```python
from build123d import *

# Parameters (mm, degrees)
SKETCH_1_W          = 147
SKETCH_1_H          = 50
SKETCH_1_R          = 1.5
EXTRUDE_1_DEPTH     = 2
CUT_EXTRUDE_1_DEPTH = 2
FILLET_2_DEPTH      = 2
FILLET_3_R          = 4
CUT_EXTRUDE_3_DEPTH = 78.661122835
SKETCH_7_R          = 1.75
CUT_EXTRUDE_4_DEPTH = 78.661122835
FILLET_4_R          = 10


with BuildPart() as part:
    # 草图1 → 凸台-拉伸1 (new body)
    with BuildSketch(Plane(origin=(0, 0, 0), x_dir=(1, 0, 0), z_dir=(0, 1, 0))):
        Rectangle(SKETCH_1_W, SKETCH_1_H)
        with Locations(Location((18, -18, 0), (0, 0, 270))):
            Circle(SKETCH_1_R, mode=Mode.SUBTRACT)
        with Locations(Location((-18, -18, 0), (0, 0, 270))):
            Circle(SKETCH_1_R, mode=Mode.SUBTRACT)
        with Locations(Location((-18, 18, 0), (0, 0, 270))):
            Circle(SKETCH_1_R, mode=Mode.SUBTRACT)
        with Locations(Location((18, 18, 0), (0, 0, 270))):
            Circle(SKETCH_1_R, mode=Mode.SUBTRACT)
    extrude(amount=EXTRUDE_1_DEPTH)

    # 草图3 → 切除-拉伸1 (cut)
    with BuildSketch(Plane(origin=(0, 2, 0), x_dir=(1, 0, 0), z_dir=(0, 1, 0))):
        with BuildLine():
            Line((-13.345416088, 16.173843213), (0, 2.828427125))
            Line((0, 2.828427125), (13.345416088, 16.173843213))
            ThreePointArc((13.345416088, 16.173843213), (13.868972045, 20.816843629), (18, 23))
            Line((18, 23), (-18, 23))
            ThreePointArc((-18, 23), (-14.464466094, 21.535533906), (-13, 18))
            ThreePointArc((-13, 18), (-13.087112888, 17.070731352), (-13.345416088, 16.173843213))
        make_face()
        with BuildLine():
            Line((16.173843213, 13.345416088), (2.828427125, 0))
            Line((2.828427125, 0), (16.173843213, -13.345416088))
            ThreePointArc((16.173843213, -13.345416088), (20.816843629, -13.868972045), (23, -18))
            Line((23, -18), (23, 18))
            ThreePointArc((23, 18), (20.816843629, 13.868972045), (16.173843213, 13.345416088))
        make_face()
        with BuildLine():
            Line((0, -2.828427125), (-13.345416088, -16.173843213))
            ThreePointArc((-13.345416088, -16.173843213), (-13.087112888, -17.070731352), (-13, -18))
            ThreePointArc((-13, -18), (-14.464466094, -21.535533906), (-18, -23))
            Line((-18, -23), (18, -23))
            ThreePointArc((18, -23), (13.868972045, -20.816843629), (13.345416088, -16.173843213))
            Line((13.345416088, -16.173843213), (0, -2.828427125))
        make_face()
        with BuildLine():
            ThreePointArc((-23, -18), (-20.816843629, -13.868972045), (-16.173843213, -13.345416088))
            Line((-16.173843213, -13.345416088), (-2.828427125, 0))
            Line((-2.828427125, 0), (-16.173843213, 13.345416088))
            ThreePointArc((-16.173843213, 13.345416088), (-20.816843629, 13.868972045), (-23, 18))
            Line((-23, 18), (-23, -18))
        make_face()
    extrude(amount=-CUT_EXTRUDE_1_DEPTH, mode=Mode.SUBTRACT)

    # 圆角2: read off the stored shape, not the designer's step
    # 圆角2 outline → 圆角2 (add)
    with BuildSketch(Plane(origin=(0, 0, 0), x_dir=(1, 0, 0), z_dir=(0, 1, 0))):
        with BuildLine():
            Line((-23, 18), (-23, 9.05572809))
            ThreePointArc((-23, 9.05572809), (-21.666666667, 12.03715206), (-18.555555556, 13.03096005))
            ThreePointArc((-18.555555556, 13.03096005), (-21.726779962, 14.666666667), (-23, 18))
        make_face()
        with BuildLine():
            ThreePointArc((-18.555555556, -13.03096005), (-21.666666667, -12.03715206), (-23, -9.05572809))
            Line((-23, -9.05572809), (-23, -18))
            ThreePointArc((-23, -18), (-21.726779962, -14.666666667), (-18.555555556, -13.03096005))
        make_face()
        with BuildLine():
            ThreePointArc((13.03096005, -18.555555556), (12.03715206, -21.666666667), (9.05572809, -23))
            Line((9.05572809, -23), (18, -23))
            ThreePointArc((18, -23), (14.666666667, -21.726779962), (13.03096005, -18.555555556))
        make_face()
        with BuildLine():
            ThreePointArc((-9.05572809, -23), (-12.03715206, -21.666666667), (-13.03096005, -18.555555556))
            ThreePointArc((-13.03096005, -18.555555556), (-14.666666667, -21.726779962), (-18, -23))
            Line((-18, -23), (-9.05572809, -23))
        make_face()
        with BuildLine():
            ThreePointArc((18.555555556, 13.03096005), (21.666666667, 12.03715206), (23, 9.05572809))
            Line((23, 9.05572809), (23, 18))
            ThreePointArc((23, 18), (21.726779962, 14.666666667), (18.555555556, 13.03096005))
        make_face()
        with BuildLine():
            ThreePointArc((23, -9.05572809), (21.666666667, -12.03715206), (18.555555556, -13.03096005))
            ThreePointArc((18.555555556, -13.03096005), (21.726779962, -14.666666667), (23, -18))
            Line((23, -18), (23, -9.05572809))
        make_face()
        with BuildLine():
            ThreePointArc((-13.03096005, 18.555555556), (-12.03715206, 21.666666667), (-9.05572809, 23))
            Line((-9.05572809, 23), (-18, 23))
            ThreePointArc((-18, 23), (-14.666666667, 21.726779962), (-13.03096005, 18.555555556))
        make_face()
        with BuildLine():
            ThreePointArc((9.05572809, 23), (12.03715206, 21.666666667), (13.03096005, 18.555555556))
            ThreePointArc((13.03096005, 18.555555556), (14.666666667, 21.726779962), (18, 23))
            Line((18, 23), (9.05572809, 23))
        make_face()
    extrude(amount=FILLET_2_DEPTH)

    # 圆角3
    fillet_3_edges = [part.edges().sort_by_distance(p)[0] for p in [
        (13.345416088, 1, 16.173843213),
        (-13.345416088, 1, 16.173843213),
        (0, 1, 2.828427125),
        (16.173843213, 1, -13.345416088),
        (16.173843213, 1, 13.345416088),
        (2.828427125, 1, 0),
        (-16.173843213, 1, -13.345416088),
        (-2.828427125, 1, 0),
        (-16.173843213, 1, 13.345416088),
        (-13.345416088, 1, -16.173843213),
        (13.345416088, 1, -16.173843213),
        (0, 1, -2.828427125),
    ]]
    fillet(fillet_3_edges, radius=FILLET_3_R)

    # 草图6 → 切除-拉伸3 (cut, through all)
    with BuildSketch(Plane(origin=(0, 2, 0), x_dir=(1, 0, 0), z_dir=(0, 1, 0))):
        Polygon((63.5, -25), (56.57179677, -13), (36.57179677, -13), (29.643593539, -25), align=None)
    cut_extrude_3 = extrude(amount=-CUT_EXTRUDE_3_DEPTH, mode=Mode.SUBTRACT)

    # 镜向1: 切除-拉伸3 across plane
    add(cut_extrude_3.mirror(Plane(origin=(0, 0, 0), x_dir=(0, 0, 1), z_dir=(1, 0, 0))), mode=Mode.SUBTRACT)

    # 草图7 → 切除-拉伸4 (cut, through all)
    with BuildSketch(Plane.XZ):
        with Locations(Location((70.5, 20, 0), (0, 0, 270))):
            Circle(SKETCH_7_R)
        with Locations(Location((70.5, -15, 0), (0, 0, 270))):
            Circle(SKETCH_7_R)
        with Locations(Location((-70.5, -15, 0), (0, 0, 270))):
            Circle(SKETCH_7_R)
        with Locations(Location((-70.5, 20, 0), (0, 0, 270))):
            Circle(SKETCH_7_R)
    extrude(amount=-CUT_EXTRUDE_4_DEPTH, mode=Mode.SUBTRACT)

    # 圆角4
    fillet_4_edges = [part.edges().sort_by_distance(p)[0] for p in [
        (63.5, 1, 25),
        (29.643593539, 1, 25),
        (36.57179677, 1, 13),
        (56.57179677, 1, 13),
        (-29.643593539, 1, 25),
        (-63.5, 1, 25),
        (-56.57179677, 1, 13),
        (-36.57179677, 1, 13),
    ]]
    fillet(fillet_4_edges, radius=FILLET_4_R)


solid = part.part
```
Verification items for the finished model (mm, model axes). A direction names the side the tool comes from. Coordinates: 2 decimals unless noted, no trailing zeros. Loops run counter-clockwise (first coordinate to the right, second up) from the corner with the lowest first, then second, coordinate; pieces in that order, holes last. Notation, with made-up numbers: (-40, 21) - (2, 21) arc R28 ccw to (2, 41) - close; hole circle Ø4 at (23.5, 87.5). An arc over 180 degrees is marked (long way). Answer as a JSON object with one key per item and string values.
(1) Cross-section at B-B, the plane x = 47. Record the boundary of the cut face in (y, z).
Response:
{"outline": "(0, -25) - (2, -25) - (2, 13) - (0, 13) - close"}
(2) Mould release check, pull along Z, two halves, no side actions. Record for faces 1 (the cylindrical face through (12.006, 0.986, -21.702)), 2 (the cylindrical face through (37.409, 0.986, 14.303)), 3 (the flat face through (-1, 2, 0)): pulls with the +Z half, pulls with the -Z half, needs draft (parallel to the pull), parting line crosses it, or undercut.
Response:
{"face 1": "undercut", "face 2": "pulls with the +Z half", "face 3": "needs draft"}
(3) Cross-section at A-A, the plane x = 7.5. Record the boundary of the cut face in (y, z).
Response:
{"outline": "(0, -25) - (2, -25) - (2, -23) - (0, -23) - close; (0, -10.33) - (2, -10.33) - (2, -4.67) - (0, -4.67) - close; (0, 4.67) - (2, 4.67) - (2, 10.33) - (0, 10.33) - close; (0, 23) - (2, 23) - (2, 25) - (0, 25) - close"}
(4) Access from +Z, -Z, +X, -X, +Y, -Y to the whole of each face (thin tool, end or side, straight path). Record for faces 4 (the cylindrical face through (-12.006, 0.986, 21.702)), 5 (the cylindrical face through (64.34, 0.99, 23.7)).
Response:
{"face 4": "+Y, -Y", "face 5": "+Z, +Y, -Y"}
(5) Go/stop test with flat-tipped pins: pin 1 Ø1 at (x, y) = (45, 1.5) entering from +Z; pin 2 Ø3 at (x, z) = (70.5, -15) entering from -Y. Record where each tip stops, or that it passes through.
Response:
{"pin 1": "stops at z = 13", "pin 2": "passes through"}
(6) Cross-section at C-C, the plane y = 0.7. Count the separate pieces of the cut face and the enclosed holes in it, then the cut area to 3 significant figures.
Response:
{"separate pieces": "1", "enclosed holes": "12", "area": "5,260 mm²"}
(7) Scan lines: line 1 along Z through (x, y) = (70.5, 1.15); line 2 along X through (y, z) = (0.25, 2); line 3 along X through (y, z) = (1.05, 10). Record each from-to range of solid material in increasing order.
Response:
{"line 1": "z = -25 to -16.75, -13.25 to 18.25, 21.75 to 25", "line 2": "x = -73.5 to -23, -5.02 to 5.02, 23 to 73.5", "line 3": "x = -73.5 to -22.89, -12.83 to -7.17, 7.17 to 12.83, 22.89 to 73.5"}
